Source: three-view drawing plus pictorial views. Frame: mm from the lowest corner of the part. Give positions to 0.01 mm unless a question says otherwise; leave off trailing zeros. Loops run counter-clockwise (first coordinate to the right, second up) from the corner with the lowest first, then second, coordinate; pieces in that order, holes last. Notation, with made-up numbers: (29, 56) -> (64, 56) arc R11 ccw to (64, 69) -> close; hole circle Ø11 at (-16.75, 75). An arc over 180 degrees is marked (long way). Put each result on its own line as item: value.
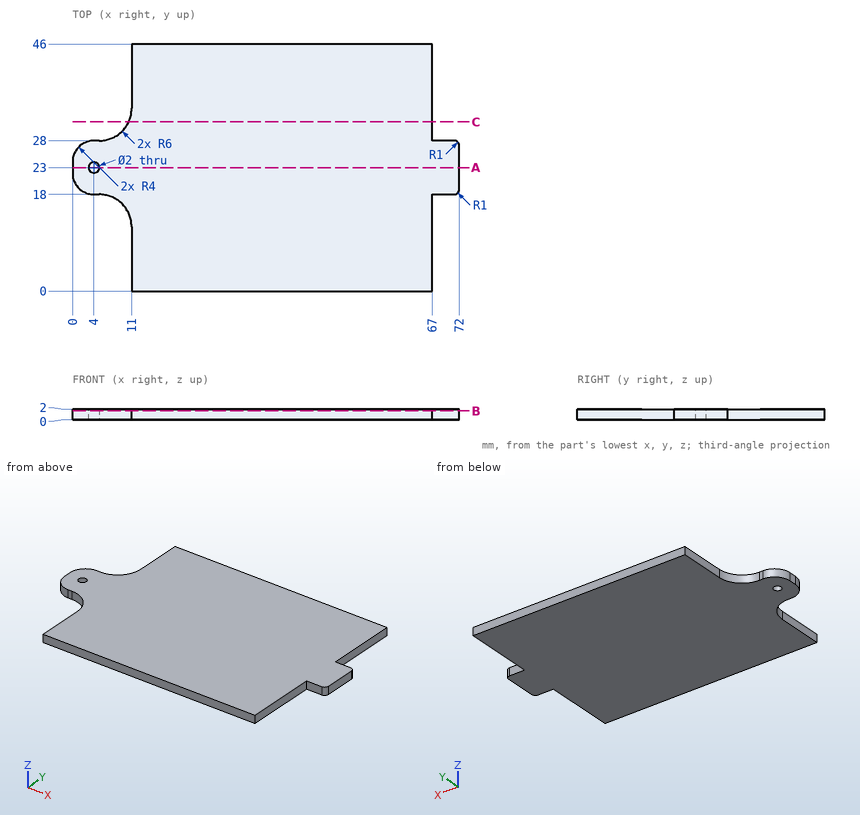
(1) Section A-A on y = 23. Return loops of the section in (x, z), then the cut area to 3 significant figures.
Calculated:
outline: (0, 0) -> (3, 0) -> (3, 2) -> (0, 2) -> close; (5, 0) -> (72, 0) -> (72, 2) -> (5, 2) -> close
area: 140 mm²
(2) Section B-B on z = 1.7. Return loops of the section in (x, y).
Calculated:
outline: (0, 22) arc R4 ccw to (4, 18) -> (5, 18) arc R6 cw to (11, 12) -> (11, 0) -> (67, 0) -> (67, 18) -> (71, 18) arc R1 ccw to (72, 19) -> (72, 27) arc R1 ccw to (71, 28) -> (67, 28) -> (67, 46) -> (11, 46) -> (11, 34) arc R6 cw to (5, 28) -> (4, 28) arc R4 ccw to (0, 24) -> close; hole circle Ø2 at (4, 23)
(3) Line query: probe 1 along Y at (x, z) = (4, 0.55); probe 2 along X at (y, z) = (9, 1.65); probe 3 along X at (y, z) = (23.5, 1.65). Output: solid intervals per line, ascending. Write a range as from..to.
Calculated:
probe 1: y = 18..22, 24..28
probe 2: x = 11..67
probe 3: x = 0..3.13, 4.87..72
(4) First-contact query: P1, Ø0.6, axis at x = 69.5, z = 0.5, coming from the -Y side; P2, Ø0.6, axis at x = 68.5, z = 1.5, coming from the +Y side; P3, Ø1, axis at y = 4.5, z = 0.5, coming from the -X side. Flat tips, straight axial feed; report the tip coordinate or a pass-through.
Calculated:
P1: stops at y = 18
P2: stops at y = 28
P3: stops at x = 11
(5) Section C-C on y = 31.5. Return loops of the section in (x, z), then the cut area to 3 significant figures.
Calculated:
outline: (10.45, 0) -> (67, 0) -> (67, 2) -> (10.45, 2) -> close
area: 113 mm²
